Here's how the part is built. I have some questions about the finished solid (model axes, mm). A direction names the side the tool comes from. Give positions to 0.01 mm unless a question says otherwise; leave off trailing zeros. Order: outer loops, then holes, each group sorted by start corner. A loop starts at its lowest first (then second) coordinate and runs counter-clockwise, first axis right, second up. Notation, with made-up numbers: (65, 28.25) -> (113, 28.25) arc R23 cw to (113, 56.25) -> close; hole circle Ø1 at (45.25, 78.5). An arc over 180 degrees is marked (long way). Write each question's results on one line, items separated by ' | '. Start each with the question number.
Q1. Imagine slicing it at A-A, the plane y = 58.5. Please give me the cut outline in (x, z).
Q2. Thinking about a two-plate mould opening in Y: for faces 1 (the face through (-2, 59, -12.5)), 2 (the face through (-3.124, 32, -31)), 3 (the face through (-2, -5, -27)), which applies, pulls with the +Y half, pulls with the -Y half, needs draft (parallel to the pull), parting line crosses it, or undercut?
Q3. I need wall thicknesses on line 1 along Z through (x, y) = (-1.85, 68); line 2 along Z through (x, y) = (-1.15, 66.5); line 3 along Y through (x, z) = (-1.2, -55). Which ranges of each line are inside material? Lowest first, please. Write a range as [from, to].
Q4. I'm going to push flat-ended pins straight in: pin 1 (0.9 mm diameter, centred on x = -1, y = -3.5, fed in from -Z); pin 2 (0.9 mm diameter, centred on x = -1.5, y = 64, fed in from +Z); pin 3 (1 mm diameter, centred on x = -2.5, z = -50, fed in from +Y). Where does each tip first touch, or does it pass through?
Q5. Imagine slicing it at B-B, the plane y = 47. Please give me the cut outline in (x, z).
Q6. For faces 4 (the face through (-2, 62, -50)), 5 (the face through (-2, 66, -49.5)), 6 (the face through (-2, 4, -46.5)), 7 (the face through (-2, 72, -45.127)), which set-ups out of +Z, -Z, +X, -X, +Y, -Y let a thin tool reach every point of the face, with its end or its side?
Q7. Imagine slicing it at C-C, the plane z = -8. Please give me the cut outline in (x, y), then the cut area to 3 significant figures.
Autodesk Inventor part; units mm, degrees
ref_plane "YZ Plane" through (0, 0, 0) normal (1, 0, 0) x (0, 1, 0)
ref_plane "XZ Plane" through (0, 0, 0) normal (0, 1, 0) x (-1, 0, 0)
ref_plane "XY Plane" through (0, 0, 0) normal (0, 0, 1) x (1, 0, 0)
sketch "Sketch3" plane through (0, 0, 0) normal (0, 1, 0) x (-1, 0, 0)
  line L0 (0, 0) -> (0, -64.031)
  line L1 (0, -64.031) -> (3.1235, -60.1267)
  line L2 (0, -64.031) -> (3.1235, -60.1267)
  line L3 (3.1235, -60.1267) -> (3.1235, -2.4988)
  line L4 (0, 0) -> (3.1235, -2.4988)
  line L5 (3.1235, -2.4988) -> (0, -2.4988)
  line L6 (0, -2.4988) -> (0, -12.4988)
  line L7 (3.1235, -2.4988) -> (3.1235, -12.4988)
  line L8 (3.1235, -60.1267) -> (0, -60.1267)
  line L9 (3.1235, -60.1267) -> (3.1235, -50.1267)
  line L10 (0, 0) -> (0, -20)
  line L11 (0, -64.031) -> (0, -48.031)
  line L12 (0, -50.1267) -> (0, -48.031)
  line L13 (0, -20) -> (0, -30)
  line L14 (0, -60.1267) -> (0, -45.1267)
  line L15 (0, -45.1267) -> (3.1235, -45.1267)
  line L16 (0, -45.1267) -> (0, -35.1267)
  line L17 (0, -35.1267) -> (3.1235, -35.1267)
  line L18 (0, -2.4988) -> (0, -22.4988)
  line L19 (0, -22.4988) -> (3.1235, -22.4988)
  line L20 (0, -22.4988) -> (0, -32.4988)
  line L21 (0, -32.4988) -> (3.1235, -32.4988)
  line L22 (0, 0) -> (0, -16)
  line L23 (0, -16) -> (3.1235, -16)
  line L24 (0, -64.031) -> (0, -48.031)
  line L25 (0, -48.031) -> (3.1235, -48.031)
  line L26 (0, -48.031) -> (0, -45.1267)
  line L27 (3.1235, -22.4988) -> (3.1235, -16)
  line L28 (3.1235, -2.4988) -> (3.1235, -1.1988)
  line L29 (3.1235, -1.1988) -> (0, 1.3)
  line L30 (0, 1.3) -> (0, 0)
  point P0 (3.1235, -20)
  point P1 (3.1235, -30)
  dimension "d80" = 15
  dimension "d81" = 10
  dimension "d86" = 20
  dimension "d87" = 10
  dimension "d90" = 16
  dimension "d91" = 16
  dimension "d92" = 2.9043
  dimension "d93" = 6.4988
  dimension "d96" = 1.3
extrude "Extrusion4" add sketch "Sketch3" along normal blind 70 contours L4 L5 L0 | L5 L3 L23 L0 | L23 L3 L19 L0 | L3 L21 L0 L19 | L3 L17 L0 L21 | L3 L15 L0 L17 | L3 L25 L0 L15 | L3 L8 L0 L25 | L1 L0 L8
sketch "Sketch4" plane through (0, 0, 0) normal (1, 0, 0) x (0, 0, -1)
  line L0 (0, 0) -> (16, 0)
  line L1 (16, 0) -> (48, 0)
  line L2 (48, 0) -> (64, 0)
  line L3 (16, 0) -> (14.5, 0)
  line L4 (14.5, 0) -> (14.5, 8)
  line L5 (14.5, 8) -> (12.5, 8)
  line L6 (12.5, 8) -> (12.5, 13)
  line L7 (12.5, 13) -> (19.5, 13)
  line L8 (19.5, 13) -> (19.5, 8)
  line L9 (19.5, 8) -> (17.5, 8)
  line L10 (16, 0) -> (17.5, 0)
  line L11 (17.5, 0) -> (17.5, 8)
  line L12 (48, 0) -> (49.5, 0)
  line L13 (48, 0) -> (46.5, 0)
  line L14 (48, 0) -> (46.5, 0)
  line L15 (46.5, 0) -> (46.5, 8)
  line L16 (46.5, 8) -> (44.5, 8)
  line L17 (44.5, 8) -> (44.5, 13)
  line L18 (44.5, 13) -> (51.5, 13)
  line L19 (51.5, 13) -> (51.5, 8)
  line L20 (51.5, 8) -> (49.5, 8)
  line L21 (49.5, 8) -> (49.5, 0)
  line L22 (16, 13) -> (16, 57)
  line L23 (16, 70) -> (17.5, 70)
  line L24 (17.5, 70) -> (17.5, 62)
  line L25 (17.5, 62) -> (19.5, 62)
  line L26 (19.5, 62) -> (19.5, 57)
  line L27 (19.5, 57) -> (12.5, 57)
  line L28 (12.5, 57) -> (12.5, 62)
  line L29 (12.5, 62) -> (14.5, 62)
  line L30 (14.5, 62) -> (14.5, 70)
  line L31 (48, 13) -> (48, 57)
  line L32 (48, 70) -> (49.5, 70)
  line L33 (49.5, 70) -> (49.5, 62)
  line L34 (49.5, 62) -> (51.5, 62)
  line L35 (51.5, 62) -> (51.5, 57)
  line L36 (51.5, 57) -> (44.5, 57)
  line L37 (44.5, 57) -> (44.5, 62)
  line L38 (44.5, 62) -> (46.5, 62)
  line L39 (46.5, 62) -> (46.5, 70)
  line L40 (46.5, 70) -> (48, 70)
  line L41 (16, 70) -> (14.5, 70)
  dimension "d23" = 16
  dimension "d24" = 32
  dimension "d25" = 16
  dimension "d26" = 1.5
  dimension "d27" = 8
  dimension "d28" = 2
  dimension "d29" = 5
  dimension "d30" = 7
  dimension "d31" = 2
  dimension "d32" = 1.5
  dimension "d33" = 1.5
  dimension "d34" = 1.5
  dimension "d35" = 1.5
  dimension "d36" = 8
  dimension "d37" = 2
  dimension "d38" = 7
  dimension "d39" = 70
  dimension "d40" = 8
  dimension "d41" = 2
  dimension "d42" = 5
  dimension "d43" = 7
  dimension "d44" = 5
  dimension "d45" = 1.5
  dimension "d46" = 8
  dimension "d47" = 2
extrude "Extrusion5" cut sketch "Sketch4" against normal blind 3.2 contours L4 L5 L6 L7 L8 L9 L11 L1 L0
extrude "Extrusion6" cut sketch "Sketch4" against normal blind 3.2 contours L15 L16 L17 L18 L19 L20 L21 L2 L1
extrude "Extrusion7" cut sketch "Sketch4" against normal blind 3.2 contours L36 L37 L38 L39 L40 L32 L33 L34 L35
extrude "Extrusion8" cut sketch "Sketch4" against normal blind 3.2 contours L27 L28 L29 L30 L41 L23 L24 L25 L26
sketch "Sketch6" plane through (0, 70, 0) normal (0, 1, 0) x (1, 0, 0)
  line L0 (0, 0) -> (0, 2.499)
  line L1 (-3.123, 2.499) -> (-3.123, 12.499)
  line L2 (0, 12.499) -> (0, 2.499)
  line L3 (0, 0) -> (0, 64)
  line L4 (0, 2.499) -> (0, 60.127)
  line L5 (-3.123, 55.127) -> (-3.123, 45.127)
  line L6 (-3.123, 55.127) -> (-3.123, 40.127)
  line L7 (-3.123, 40.127) -> (-3.123, 30.127)
  line L8 (0, 30.127) -> (0, 40.127)
  line L9 (-3.123, 60.127) -> (0, 60.127)
  line L10 (-3.123, 60.127) -> (-3.123, 45.127)
  line L11 (-3.123, 45.127) -> (0, 45.127)
  line L12 (-3.123, 45.127) -> (-3.123, 35.127)
  line L13 (-3.123, 35.127) -> (0, 35.127)
  line L14 (0, 35.127) -> (0, 45.127)
  line L15 (-3.123, 2.499) -> (0, 2.499)
  line L16 (-3.123, 2.499) -> (-3.123, 22.499)
  line L17 (-3.123, 22.499) -> (0, 22.499)
  line L18 (-3.123, 22.499) -> (-3.123, 32.499)
  line L19 (-3.123, 32.499) -> (0, 32.499)
  line L20 (0, 32.499) -> (0, 22.499)
  line L21 (-3.123, 2.3854) -> (-3.123, 1.3854)
  line L22 (-2.9831, 1.2495) -> (0, -1.1378)
  line L23 (-2.9831, 1.2495) -> (0.8377, 1.2495) construction
  line L24 (0, -1.1378) -> (0, 0)
  dimension "d63" = 3.123
  dimension "d65" = 64
  dimension "d75" = 15
  dimension "d76" = 10
  dimension "d77" = 20
  dimension "d78" = 10
  dimension "d94" = 1
  dimension "d95" = 38.67
extrude "Extrusion13" add sketch "Sketch6" along normal blind 5 contours L18 L7 L19 L3 L17 | L7 L6 L11 L3 L13
extrude "Extrusion14" add sketch "Sketch3" against normal blind 5 contours L3 L21 L0 L19 | L3 L15 L0 L17
extrude "Extrusion15" add sketch "Sketch3" along normal blind 70 contours L30 L29 L28 L4
properties part number "lat_front_mdf"
Geometry check:
1) outline: (-3.12, -60.13) -> (0, -64.03) -> (0, -51.5) -> (-3.12, -51.5) -> close; (-3.12, -44.5) -> (0, -44.5) -> (0, -19.5) -> (-3.12, -19.5) -> close; (-3.12, -12.5) -> (0, -12.5) -> (0, 1.3) -> (-3.12, -1.2) -> close
2) face 1: undercut | face 2: needs draft | face 3: pulls with the -Y half
3) line 1: [-61.72, -49.5], [-46.5, -17.5], [-14.5, -0.18] | line 2: [-62.59, -49.5], [-46.5, -17.5], [-14.5, 0.38] | line 3: [0, 70]
4) pin 1: z = -45.13 | pin 2: z = 0.46 | pin 3: y = 70
5) outline: (-3.12, -60.13) -> (0, -64.03) -> (0, 1.3) -> (-3.12, -1.2) -> close
6) face 4: +X, -X | face 5: +X, -X, +Y | face 6: +X, -X, -Y | face 7: -Z, +X, -X, +Y
7) outline: (-3.12, 0) -> (0, 0) -> (0, 70) -> (-3.12, 70) -> close | area: 219 mm²
